The listing builds one solid part. Answer for the finished solid, in the listing's coordinates (mm). Face numbers are marked on the shaded views. A direction names the side the tool comes from. Round coordinates to 2 decimals unless told otherwise and drop trailing zeros. Loops run counter-clockwise (first coordinate to the right, second up) from the corner with the lowest first, then second, coordinate; pieces in that order, holes last. Notation, with made-up numbers: (10.5, 62) -> (34.5, 62) arc R35 ccw to (34.5, 98) -> close; hole circle Ø11 at (69, 26.5). An arc over 180 degrees is marked (long way). Write each question's results on one line, items separated by ' | '. Start each with the question number.
(1) The part is cut by section C-C (x = 43). Determine the outline of the cut face in (y, z), plus the area to 3 significant figures.
(2) Determine the mould class of the marked faces 1, 2 and 3 for opening direction Y: released by +Y, released by -Y, zero draft, split by the parting line, or undercut.
(3) For the marked faces 4, 5, 6 and 7, determine the directions among +Z, -Z, +X, -X, +Y, -Y from which every point of the face is accessible in a straight line to the end or side of a thin tool.
(4) The part is cut by section A-A (x = 0). Determine the outline of the cut face in (y, z).
(5) The part is cut by section B-B (y = 4). Determine the outline of the cut face in (x, z), plus the area to 3 significant figures.
(6) The part is cut by section D-D (z = 5.75). Determine the outline of the cut face in (x, y).
(7) Flat-ended cylindrical pins translate along their axes: pin 1 (1.5 mm diameter, centred on y = -5, z = 5.5, fed in from +X) (3 decimals); pin 2 (4 mm diameter, centred on y = 38.5, z = 5.5, fed in from -X); pin 3 (1 mm diameter, centred on y = -1, z = 1.5, fed in from +X). Find the tip coordinate at first contact, or state that the pin passes through.
(8) Straight lines are drawn through the part: probe 1 along X at (y, z) = (29.5, 4.75); probe 2 along X at (y, z) = (40, 2.5); probe 3 along X at (y, z) = (34.5, 4.25). For each, find the intervals that lie inside material, in ascending order.
```python
from build123d import *

# Parameters (mm, degrees)
F1_R      = 22.86
F8_DEPTH  = 8.382
F5_R      = 22.86
F5_R_2    = 23.2590602535
F5_R_3    = 22.8896939672
F3_R      = 12.065
F9_DEPTH  = 25.908
F0_R      = 12.065
F10_DEPTH = 39.878
F12_R     = 12.0825397837
F12_R_2   = 12.1193647321
F12_R_3   = 12.0891778509
F13_DEPTH = 25.4
F14_R     = 12.3194510373
F15_DEPTH = 25.4


with BuildPart() as f8:
    # F1 (on Top) → F8 (new body)
    with BuildSketch(Plane.XY):
        Circle(F1_R)
    extrude(amount=F8_DEPTH)

    # F3 (on Top) → F9 (cut)
    with BuildSketch(Plane.XY):
        with Locations((-41.2355296061, 30.9968510523)):
            Circle(F3_R)
        with Locations((47.3912737196, 20.2672132623)):
            Circle(F3_R)
        with Locations((-6.2569124064, -50.5483931394)):
            Circle(F3_R)
    extrude(amount=-F9_DEPTH, mode=Mode.SUBTRACT)


with BuildPart() as f8b:
    # F4 (on Top) → F8, piece 2 (new body)
    with BuildSketch(Plane.XY):
        Polygon((-7.2568234486, -9.9568761684), (0, 0), (-40.8516675234, 30.6916665286), (-48.2515008219, 20.8422329908), align=None)
        Polygon((-40.8516675234, 30.6916665286), (0, 0), (6.6820263642, 9.1682138243), (-33.8416725592, 39.6134790794), align=None)
    extrude(amount=F8_DEPTH)


with BuildPart() as f8c:
    # F5 (on Top) → F8, piece 3 (new body)
    with BuildSketch(Plane.XY):
        with Locations((-41.0204199318, 30.6730984167)):
            Circle(F5_R)
    extrude(amount=F8_DEPTH)


with BuildPart() as f8d:
    # F5 (on Top) → F8, piece 4 (new body)
    with BuildSketch(Plane.XY):
        with Locations((46.5983533047, 20.1435375921)):
            Circle(F5_R_2)
    extrude(amount=F8_DEPTH)


with BuildPart() as f8e:
    # F5 (on Top) → F8, piece 5 (new body)
    with BuildSketch(Plane.XY):
        with Locations((-6.2648058406, -49.9444669655)):
            Circle(F5_R_3)
    extrude(amount=F8_DEPTH)


with BuildPart() as f8f:
    # F6 (on Top) → F8, piece 6 (new body)
    with BuildSketch(Plane.XY):
        Polygon((-6.1354051676, -50.8), (0, 0), (-12.4105271356, 2.6960742232), (-18.6884442668, -49.2838980126), align=None)
        Polygon((12.7, -1.5338512919), (0, 0), (-6.1354051676, -50.8), (6.5645948324, -52.3338512919), align=None)
    extrude(amount=F8_DEPTH)


with BuildPart() as f8g:
    # F7 (on Top) → F8, piece 7 (new body)
    with BuildSketch(Plane.XY):
        Polygon((-4.6202341585, 10.9058370142), (0, 0), (46.7755481242, 19.8163593447), (41.3952207145, 32.5163593447), align=None)
        Polygon((46.7755481242, 19.8163593447), (0, 0), (5.4993537205, -11.462887171), (51.7296379604, 8.1224723137), align=None)
    extrude(amount=F8_DEPTH)


with BuildPart() as f10_tool:
    # F0 (on Top) → F10 (new body)
    with BuildSketch(Plane.XY):
        Circle(F0_R)
    extrude(amount=F10_DEPTH)


with BuildPart() as f8_1:
    add(f8.part)

    # F10: cut by f10_tool
    add(f10_tool.part, mode=Mode.SUBTRACT)


with BuildPart() as f8b_1:
    add(f8b.part)

    # F10: cut by f10_tool
    add(f10_tool.part, mode=Mode.SUBTRACT)


with BuildPart() as f8f_1:
    add(f8f.part)

    # F10: cut by f10_tool
    add(f10_tool.part, mode=Mode.SUBTRACT)


with BuildPart() as f8g_1:
    add(f8g.part)

    # F10: cut by f10_tool
    add(f10_tool.part, mode=Mode.SUBTRACT)


with BuildPart() as f8f_2:
    add(f8f_1.part)

    # F11: union F8b, F8c, F8, F8d, F8e, F8g
    add(f8b_1.part)
    add(f8c.part)
    add(f8_1.part)
    add(f8d.part)
    add(f8e.part)
    add(f8g_1.part)

    # F12 (on face) → F13 (cut)
    with BuildSketch(Plane.XY.offset(8.382)):
        with Locations((-41.0204199318, 30.6730984167)):
            Circle(F12_R)
        with Locations((-6.2648058406, -49.9444669655)):
            Circle(F12_R_2)
        with Locations((46.5983533047, 20.1435375921)):
            Circle(F12_R_3)
    extrude(amount=-F13_DEPTH, mode=Mode.SUBTRACT)

    # F14 (on face) → F15 (cut)
    with BuildSketch(Plane(origin=(0, 0, 0), x_dir=(1, 0, 0), z_dir=(0, 0, -1))):
        Circle(F14_R)
    extrude(amount=-F15_DEPTH, mode=Mode.SUBTRACT)


solid = f8f_2.part
```
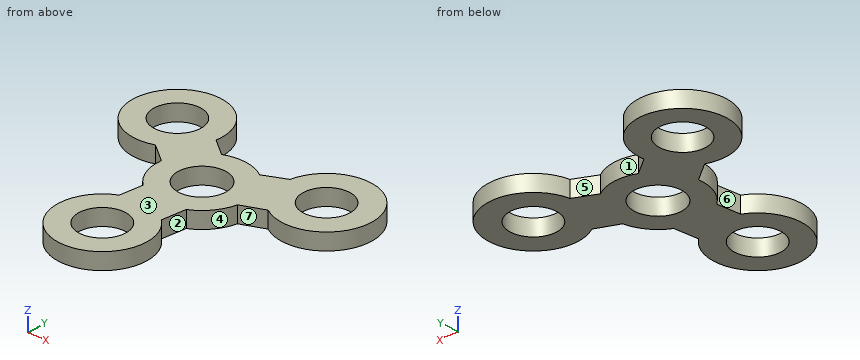
Checked values:
1) outline: (-2.84, 0) -> (8.6, 0) -> (8.6, 8.38) -> (-2.84, 8.38) -> close; (31.68, 0) -> (43.12, 0) -> (43.12, 8.38) -> (31.68, 8.38) -> close | area: 192 mm2
2) face 1: released by +Y | face 2: undercut | face 3: zero draft
3) face 4: +Z, -Z, +X | face 5: +Z, -Z, +Y | face 6: +Z, -Z, -X | face 7: +Z, -Z, -Y
4) outline: (-71.96, 0) -> (-60.32, 0) -> (-60.32, 8.38) -> (-71.96, 8.38) -> close; (-39.57, 0) -> (-12.32, 0) -> (-12.32, 8.38) -> (-39.57, 8.38) -> close; (12.32, 0) -> (22.86, 0) -> (22.86, 8.38) -> (12.32, 8.38) -> close
5) outline: (-25.83, 0) -> (-11.65, 0) -> (-11.65, 8.38) -> (-25.83, 8.38) -> close; (11.65, 0) -> (63.34, 0) -> (63.34, 8.38) -> (11.65, 8.38) -> close | area: 552 mm2
6) outline: (-32.9, 9.31) -> (-22.8, 1.72) arc R22.86 ccw to (-14.84, -17.39) -> (-16.28, -29.36) arc R22.89 ccw (long way) to (8.92, -32.82) -> (10.43, -20.34) arc R22.86 ccw to (22.46, -4.28) -> (33.98, 0.6) arc R23.26 ccw (long way) to (23.7, 24.2) -> (12.67, 19.03) arc R22.86 ccw to (-9.05, 20.99) -> (-18.32, 27.95) arc R22.86 ccw (long way) to start; hole circle Ø24.17 at (-41.02, 30.67); hole circle Ø24.24 at (-6.26, -49.94); hole circle Ø24.64 at (0, 0); hole circle Ø24.18 at (46.6, 20.14)
7) pin 1: stops at x = 22.525 | pin 2: stops at x = -63.13 | pin 3: stops at x = 57.31
8) probe 1: x = -63.85 to -53.05, -28.99 to -18.19, 25.3 to 38.94, 54.25 to 67.89 | probe 2: x = -61.89 to -48.7, -33.34 to -20.15, 34.49 to 58.71 | probe 3: x = -63.56 to -52.48, -29.56 to -18.48, 28.3 to 64.9
